```python
from build123d import *

# Parameters (mm, degrees)
SKETCH1_W           = 104.14
SKETCH1_H           = 78.74
BOSS_EXTRUDE1_DEPTH = 19.05
SKETCH2_W           = 96.52
SKETCH2_H           = 71.12
CUT_EXTRUDE1_DEPTH  = 14.2875
CUT_EXTRUDE2_REACH  = 6.763
SKETCH4_W           = 3.81
SKETCH4_H           = 59.69
CUT_EXTRUDE3_DEPTH  = 14.2875
FILLET1_R           = 2.54
BOSS_EXTRUDE2_DEPTH = 3.175
CUT_EXTRUDE4_REACH  = 5.175
SKETCH6_R           = 2.54
FILLET2_R           = 2.54


with BuildPart() as part:
    # Sketch1 → Boss-Extrude1 (new body)
    with BuildSketch(Plane(origin=(0, 0, 0), x_dir=(1, 0, 0), z_dir=(0, 1, 0))):
        with Locations((52.07, 39.37)):
            Rectangle(SKETCH1_W, SKETCH1_H)
    extrude(amount=BOSS_EXTRUDE1_DEPTH)

    # Sketch2 → Cut-Extrude1 (cut)
    with BuildSketch(Plane(origin=(0, 19.05, 0), x_dir=(1, 0, 0), z_dir=(0, 1, 0))):
        with Locations((52.07, 39.37)):
            Rectangle(SKETCH2_W, SKETCH2_H)
    extrude(amount=-CUT_EXTRUDE1_DEPTH, mode=Mode.SUBTRACT)

    # Sketch3 → Cut-Extrude2 (cut, up to next)
    with BuildSketch(Plane(origin=(0, 4.7625, 0), x_dir=(1, 0, 0), z_dir=(0, 1, 0)), mode=Mode.PRIVATE) as cut_extrude2_sk1:
        with BuildLine():
            Line((22.86, 62.23), (81.28, 62.23))
            ThreePointArc((81.28, 62.23), (85.770128061, 60.370128061), (87.63, 55.88))
            Line((87.63, 55.88), (87.63, 22.86))
            ThreePointArc((87.63, 22.86), (85.770128061, 18.369871939), (81.28, 16.51))
            Line((81.28, 16.51), (22.86, 16.51))
            ThreePointArc((22.86, 16.51), (18.369871939, 18.369871939), (16.51, 22.86))
            Line((16.51, 22.86), (16.51, 55.88))
            ThreePointArc((16.51, 55.88), (18.369871939, 60.370128061), (22.86, 62.23))
        make_face()
    cut_extrude2_tool1 = extrude(cut_extrude2_sk1.sketch, amount=-CUT_EXTRUDE2_REACH, mode=Mode.PRIVATE) & part.part
    add(cut_extrude2_tool1.solids().sort_by_distance((52.07, 4.7625, -39.37))[0], mode=Mode.SUBTRACT)

    # Sketch4 → Cut-Extrude3 (cut)
    with BuildSketch(Plane(origin=(0, 19.05, 0), x_dir=(1, 0, 0), z_dir=(0, 1, 0))):
        with Locations((1.905, 39.37)):
            Rectangle(SKETCH4_W, SKETCH4_H)
    extrude(amount=-CUT_EXTRUDE3_DEPTH, mode=Mode.SUBTRACT)

    # Fillet1
    fillet1_edges = [part.edges().sort_by_distance(p)[0] for p in [
        (1.905, 19.05, -69.215),
        (1.905, 19.05, -9.525),
        (1.905, 4.7625, -69.215),
        (1.905, 4.7625, -9.525),
    ]]
    fillet(fillet1_edges, radius=FILLET1_R)

    # Sketch5 → Boss-Extrude2 (add)
    with BuildSketch(Plane.XZ):
        with BuildLine():
            Line((97.79, 0), (85.09, 0))
            Line((85.09, 0), (85.09, 19.685))
            ThreePointArc((85.09, 19.685), (85.833948776, 21.481051224), (87.63, 22.225))
            Line((87.63, 22.225), (95.25, 22.225))
            ThreePointArc((95.25, 22.225), (97.046051224, 21.481051224), (97.79, 19.685))
            Line((97.79, 19.685), (97.79, 0))
        make_face()
        with BuildLine():
            Line((85.09, -78.74), (85.09, -98.425))
            ThreePointArc((85.09, -98.425), (85.833948776, -100.221051224), (87.63, -100.965))
            Line((87.63, -100.965), (95.25, -100.965))
            ThreePointArc((95.25, -100.965), (97.046051224, -100.221051224), (97.79, -98.425))
            Line((97.79, -98.425), (97.79, -78.74))
            Line((97.79, -78.74), (85.09, -78.74))
        make_face()
        with BuildLine():
            Line((12.7, 0), (25.4, 0))
            Line((25.4, 0), (25.4, 50.8))
            ThreePointArc((25.4, 50.8), (24.656051224, 52.596051224), (22.86, 53.34))
            Line((22.86, 53.34), (15.24, 53.34))
            ThreePointArc((15.24, 53.34), (13.443948776, 52.596051224), (12.7, 50.8))
            Line((12.7, 50.8), (12.7, 0))
        make_face()
        with BuildLine():
            Line((25.4, -78.74), (25.4, -129.54))
            ThreePointArc((25.4, -129.54), (24.656051224, -131.336051224), (22.86, -132.08))
            Line((22.86, -132.08), (15.24, -132.08))
            ThreePointArc((15.24, -132.08), (13.443948776, -131.336051224), (12.7, -129.54))
            Line((12.7, -129.54), (12.7, -78.74))
            Line((12.7, -78.74), (25.4, -78.74))
        make_face()
    extrude(amount=-BOSS_EXTRUDE2_DEPTH)

    # Sketch6 → Cut-Extrude4 (cut, up to next)
    with BuildSketch(Plane(origin=(0, 3.175, 0), x_dir=(1, 0, 0), z_dir=(0, 1, 0)), mode=Mode.PRIVATE) as cut_extrude4_sk1:
        with Locations((19.05, 127)):
            Circle(SKETCH6_R)
    cut_extrude4_tool1 = extrude(cut_extrude4_sk1.sketch, amount=-CUT_EXTRUDE4_REACH, mode=Mode.PRIVATE) & part.part
    add(cut_extrude4_tool1.solids().sort_by_distance((19.05, 3.175, -127))[0], mode=Mode.SUBTRACT)
    # Sketch6 → Cut-Extrude4 (cut, up to next)
    with BuildSketch(Plane(origin=(0, 3.175, 0), x_dir=(1, 0, 0), z_dir=(0, 1, 0)), mode=Mode.PRIVATE) as cut_extrude4_sk2:
        with Locations((19.05, -48.26)):
            Circle(SKETCH6_R)
    cut_extrude4_tool2 = extrude(cut_extrude4_sk2.sketch, amount=-CUT_EXTRUDE4_REACH, mode=Mode.PRIVATE) & part.part
    add(cut_extrude4_tool2.solids().sort_by_distance((19.05, 3.175, 48.26))[0], mode=Mode.SUBTRACT)
    # Sketch6 → Cut-Extrude4 (cut, up to next)
    with BuildSketch(Plane(origin=(0, 3.175, 0), x_dir=(1, 0, 0), z_dir=(0, 1, 0)), mode=Mode.PRIVATE) as cut_extrude4_sk3:
        with Locations((91.44, -17.145)):
            Circle(SKETCH6_R)
    cut_extrude4_tool3 = extrude(cut_extrude4_sk3.sketch, amount=-CUT_EXTRUDE4_REACH, mode=Mode.PRIVATE) & part.part
    add(cut_extrude4_tool3.solids().sort_by_distance((91.44, 3.175, 17.145))[0], mode=Mode.SUBTRACT)
    # Sketch6 → Cut-Extrude4 (cut, up to next)
    with BuildSketch(Plane(origin=(0, 3.175, 0), x_dir=(1, 0, 0), z_dir=(0, 1, 0)), mode=Mode.PRIVATE) as cut_extrude4_sk4:
        with Locations((91.44, 95.885)):
            Circle(SKETCH6_R)
    cut_extrude4_tool4 = extrude(cut_extrude4_sk4.sketch, amount=-CUT_EXTRUDE4_REACH, mode=Mode.PRIVATE) & part.part
    add(cut_extrude4_tool4.solids().sort_by_distance((91.44, 3.175, -95.885))[0], mode=Mode.SUBTRACT)

    # Fillet2
    fillet2_edges = [part.edges().sort_by_distance(p)[0] for p in [
        (91.44, 3.175, 0),
        (97.79, 1.5875, 0),
        (85.09, 1.5875, 0),
        (91.44, 3.175, -78.74),
        (85.09, 1.5875, -78.74),
        (97.79, 1.5875, -78.74),
        (12.7, 1.5875, 0),
        (19.05, 3.175, 0),
        (25.4, 1.5875, 0),
        (19.05, 3.175, -78.74),
        (12.7, 1.5875, -78.74),
        (25.4, 1.5875, -78.74),
    ]]
    fillet(fillet2_edges, radius=FILLET2_R)


solid = part.part
```
The listing builds one solid part. Answer for the finished solid, in the listing's coordinates (mm). A direction names the side the tool comes from. Round coordinates to 2 decimals unless told otherwise and drop trailing zeros. Write each loop counter-clockwise with the first axis right and the second up, starting at its lowest first coordinate (ties: lowest second). Pieces come first, ordered by that corner, then holes. Notation, with made-up numbers: (87.5, 5.5) -> (130.5, 5.5) arc R23 ccw to (130.5, 39.5) -> close; hole circle Ø5 at (-12.5, 3.25). An arc over 180 degrees is marked (long way). Answer as a JSON object with one key per item and string values. Group by question number.
Q1. Determine the mould class of faces 4 (the face through (91, 3.175, -91)), 5 (the face through (87.63, 2, -40)), 6 (the face through (18.5, 1.61, -124.52)), 7 (the face through (51, 9, -78.74)) for opening direction Z: pulls with the +Z half, pulls with the -Z half, needs draft (parallel to the pull), parting line crosses it, or undercut.
Q2. Straight lines are drawn through the part: line 1 along Z through (x, y) = (91.44, 1.85) (3 decimals); line 2 along Z through (x, y) = (9.5, 9.75); line 3 along Z through (x, y) = (19.05, 1.6). For each, find the intervals that lie inside material, in ascending order.
Q3. Section D-D (y = 11.5) is taken. Write down the section's boundary in (x, z) (3 decimals).
Q4. Section B-B (x = 77) is taken. Write down the section's boundary in (y, z).
Q5. Section A-A (z = 48.26) is taken. Write down the section's boundary in (x, y) (3 decimals), plus the area to 3 significant figures.
Q6. Which of the six approach directions +Z, -Z, +X, -X, +Y, -Y give full straight-line access (tool end or side, diameter ignored) to faces 1 (the face through (2, 12, -9.525)), 2 (the face through (3.81, 12, -72)), 3 (the face through (18.42, 2.41, -18.32))?
Q7. Section C-C (x = 19.05) is taken. Count the separate pieces of the cut face and the enclosed holes in it, plus the area to 3 significant figures.
Q8. Each of these flat-tipped pins is pushed along its axis until it touches: pin 1 Ø1.5 at (x, y) = (43, 9.5) entering from +Z; pin 2 Ø1.6 at (y, z) = (2, -109.5) entering from +X; pin 3 Ø1.6 at (y, z) = (2, 9) entering from +X; pin 4 Ø6 at (x, y) = (16, 4.5) entering from +Z. Where does it stop, or does it pass through?
Check values:
{
 "1": {"face 4": "needs draft", "face 5": "undercut", "face 6": "undercut", "face 7": "pulls with the -Z half"},
 "2": {"line 1": "-100.965 to -98.425, -93.345 to 14.605, 19.685 to 22.225", "line 2": "-78.74 to -74.93, -3.81 to 0", "line 3": "-132.08 to -129.54, -124.46 to -60.96, -17.78 to 45.72, 50.8 to 53.34"},
 "3": {"outline": "(0, -78.74) -> (104.14, -78.74) -> (104.14, 0) -> (0, 0) -> (0, -9.525) -> (3.81, -9.525) -> (3.81, -3.81) -> (100.33, -3.81) -> (100.33, -74.93) -> (3.81, -74.93) -> (3.81, -69.215) -> (0, -69.215) -> close"},
 "4": {"outline": "(0, -78.74) -> (19.05, -78.74) -> (19.05, -74.93) -> (4.76, -74.93) -> (4.76, -62.23) -> (0, -62.23) -> close; (0, -16.51) -> (4.76, -16.51) -> (4.76, -3.81) -> (19.05, -3.81) -> (19.05, 0) -> (0, 0) -> close"},
 "5": {"outline": "(12.7, 0) -> (16.51, 0) -> (16.51, 3.175) -> (12.7, 3.175) -> close; (21.59, 0) -> (25.4, 0) -> (25.4, 3.175) -> (21.59, 3.175) -> close", "area": "24.2 mm^2"},
 "6": {"face 1": "-X, +Y", "face 2": "+Y", "face 3": "+Y, -Y"},
 "7": {"separate pieces": "4", "enclosed holes": "0", "area": "587 mm^2"},
 "8": {"pin 1": "z = 0", "pin 2": "x = 25.4", "pin 3": "x = 97.79", "pin 4": "z = 53.34"}
}
